Here's how the part is built. I have some questions about the finished solid (model axes, mm). Face numbers are marked on the shaded views. A direction names the side the tool comes from. Coordinates: 2 decimals unless noted, no trailing zeros. Write each loop counter-clockwise with the first axis right and the second up, starting at its lowest first coordinate (ties: lowest second). Pieces come first, ordered by that corner, then holes.
```python
from build123d import *

# Parameters (mm, degrees)
SKETCH1_R           = 5
BOSS_EXTRUDE1_DEPTH = 10
CUT_EXTRUDE1_DEPTH  = 10
FILLET1_R           = 20


with BuildPart() as part:
    # Sketch1 → Boss-Extrude1 (new body)
    with BuildSketch(Plane(origin=(0, 0, 0), x_dir=(1, 0, 0), z_dir=(0, 1, 0))):
        with BuildLine():
            Line((43.536010052, -35.595148029), (18.411320837, 40))
            Line((18.411320837, 40), (-50, 40))
            Line((-50, 40), (-50, -13))
            Line((-50, -13), (-50, -33.474160509))
            Line((-50, -33.474160509), (-30, -33.474160509))
            Line((-30, -33.474160509), (-30, -13))
            Line((-30, -13), (10.471929596, -22.862355971))
            ThreePointArc((10.471929596, -22.862355971), (14.880225334, -25.223606168), (17.593976856, -29.424097387))
            Line((17.593976856, -29.424097387), (19.644977926, -35.595148029))
            Line((19.644977926, -35.595148029), (43.536010052, -35.595148029))
        make_face()
        Circle(SKETCH1_R, mode=Mode.SUBTRACT)
    extrude(amount=BOSS_EXTRUDE1_DEPTH)

    # Sketch2 → Cut-Extrude1 (cut)
    with BuildSketch(Plane(origin=(0, 10, 0), x_dir=(1, 0, 0), z_dir=(0, 1, 0))):
        Polygon((21.565271485, 30.510395408), (12.075666894, 27.35644476), (18.38356819, 8.377235576), (27.873172782, 11.531186225), align=None)
        Polygon((34.181074079, -7.448022959), (24.691469487, -10.601973607), (30.999370784, -29.581182791), (40.488975376, -26.427232142), align=None)
    extrude(amount=-CUT_EXTRUDE1_DEPTH, mode=Mode.SUBTRACT)

    # Fillet1
    fillet1_edges = [part.edges().sort_by_distance(p)[0] for p in [
        (-50, 5, -40),
    ]]
    fillet(fillet1_edges, radius=FILLET1_R)


solid = part.part
```
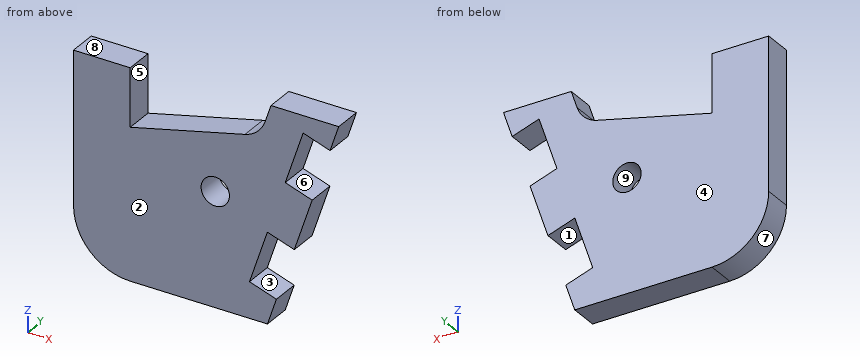
1) We'd pull the mould along Z, two halves only. Please class the marked faces 6, 7, 8 and 9: pulls with the +Z half, pulls with the -Z half, needs draft (parallel to the pull), parting line crosses it, or undercut.
Values follow:
face 6: undercut
face 7: pulls with the -Z half
face 8: pulls with the +Z half
face 9: undercut
2) Imagine slicing it at D-D on x = -11. Please give me the cut outline in (y, z).
Values follow:
outline: (0, -40) - (10, -40) - (10, 17.63) - (0, 17.63) - close
3) I need wall thicknesses on probe 1 along Z at (x, y) = (0, 4.25); probe 2 along X at (y, z) = (4.5, 0); probe 3 along Z at (x, y) = (-3, 6.25). Which ranges of each line are inside material? Lowest first, please.
Values follow:
probe 1: z = -40 to -5, 5 to 20.31
probe 2: x = -50 to -5, 5 to 31.71
probe 3: z = -40 to -4, 4 to 19.58
4) Imagine slicing it at C-C on x = 0. Please give me the cut outline in (y, z).
Values follow:
outline: (0, -40) - (10, -40) - (10, -5) - (0, -5) - close; (0, 5) - (10, 5) - (10, 20.31) - (0, 20.31) - close
5) Imagine slicing it at B-B on y = 4.5. Please give me the cut outline in (x, z).
Values follow:
outline: (-50, -20) arc R20 ccw to (-30, -40) - (18.41, -40) - (21.57, -30.51) - (12.08, -27.36) - (18.38, -8.38) - (27.87, -11.53) - (34.18, 7.45) - (24.69, 10.6) - (31, 29.58) - (40.49, 26.43) - (43.54, 35.6) - (19.64, 35.6) - (17.59, 29.42) arc R10 cw to (10.47, 22.86) - (-30, 13) - (-30, 33.47) - (-50, 33.47) - close; hole circle Ø10 at (0, 0)
6) On a 3-axis mill with a long thin cutter (end or side, diameter ignored), from which of +Z, -Z, +X, -X, +Y, -Y can I reach the whole of each face in a straight line? I mean the marked faces 1, 2, 3, 4 and 5. Say none if no direction works.
Values follow:
face 1: +Y, -Y
face 2: +Z, -Z, +X, -X, -Y
face 3: +X, +Y, -Y
face 4: +Z, -Z, +X, -X, +Y
face 5: +Z, +Y, -Y
7) Imagine slicing it at A-A on z = -3.5. Please give me the cut outline in (x, y), then the cut area to 3 significant figures.
Values follow:
outline: (-50, 0) - (-3.57, 0) - (-3.57, 10) - (-50, 10) - close; (3.57, 0) - (30.54, 0) - (30.54, 10) - (3.57, 10) - close
area: 734 mm2
8) Will these pins go through, and if not, where does the flat tip stop? pin 1 (6 mm diameter, centred on y = 4, z = -7, fed in from +X); pin 2 (3 mm diameter, centred on x = -35, y = 2.5, fed in from +Z); pin 3 (5 mm diameter, centred on x = 8, y = 3.5, fed in from +Z).
Values follow:
pin 1: stops at x = 30.38
pin 2: stops at z = 33.47
pin 3: stops at z = 22.87
